Print and shaded views of the part. All mm, measured from the part's lowest x, y and z. A direction names the side the tool comes from. Give positions to 0.01 mm unless a question says otherwise; leave off trailing zeros. Loops run counter-clockwise (first coordinate to the right, second up) from the corner with the lowest first, then second, coordinate; pieces in that order, holes last. Notation, with made-up numbers: (84, -40) - (134, -40) arc R9 ccw to (134, -33) - close; hole circle Ø5 at (47, 54). An arc over 180 degrees is marked (long way). Return JSON: item names as keys, results as strings.
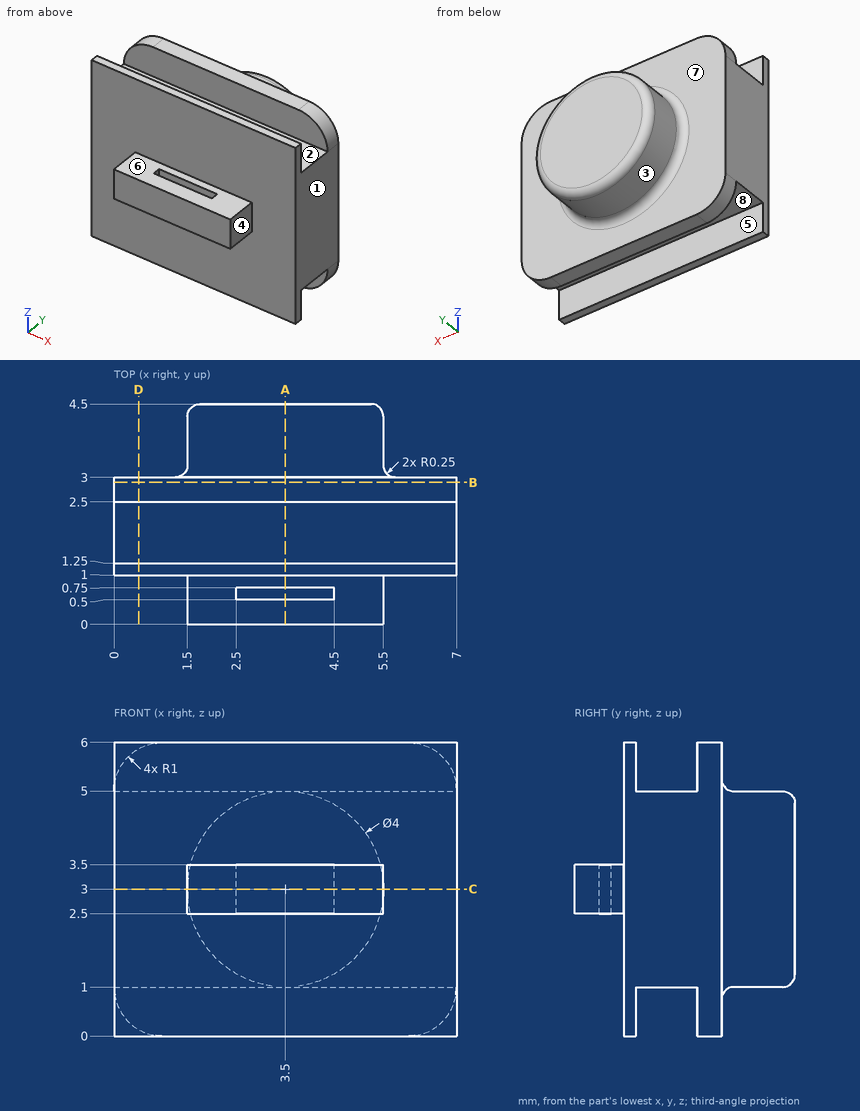
1. Drill centre lines: probe 1 along Y at (x, z) = (2.5, 5.45); probe 2 along Y at (x, z) = (4, 3); probe 3 along Y at (x, z) = (0.5, 1.8). Where is each one in solid material? Low to high.
Values follow:
{"probe 1": "y = 1 to 1.25, 2.5 to 3", "probe 2": "y = 0 to 0.5, 0.75 to 4.5", "probe 3": "y = 1 to 3"}
2. Drop flat-ended pins along their axis: P1, Ø0.8, axis at x = 2.5, y = 0.5, coming from the -Z side; P2, Ø0.8, axis at x = 3.5, y = 0.5, coming from the +Z side; P3, Ø0.5, axis at y = 0.5, z = 3, coming from the +X side. Give the stop position or say it passes through.
Values follow:
{"P1": "stops at z = 2.5", "P2": "stops at z = 3.5", "P3": "stops at x = 5.5"}
3. Which spindle directions (+Z, -Z, +X, -X, +Y, -Y) get a long thin tool onto all of the face, cutting with end or side? Do the marked faces 1, 2, 3, 4 and 5. Say none if no direction does.
Values follow:
{"face 1": "+Z, -Z, +X, +Y, -Y", "face 2": "+Z, +X, -X", "face 3": "+Y", "face 4": "+Z, -Z, +X, -Y", "face 5": "-Z, +X, -X"}
4. Cut at B-B, the plane y = 2.9. Write the cut outline in (x, z).
Values follow:
{"outline": "(0, 1) arc R1 ccw to (1, 0) - (6, 0) arc R1 ccw to (7, 1) - (7, 5) arc R1 ccw to (6, 6) - (1, 6) arc R1 ccw to (0, 5) - close"}
5. Cut at A-A, the plane x = 3.5. Write the cut outline in (y, z).
Values follow:
{"outline": "(0, 2.5) - (0.5, 2.5) - (0.5, 3.5) - (0, 3.5) - close; (0.75, 2.5) - (1, 2.5) - (1, 0) - (1.25, 0) - (1.25, 1) - (2.5, 1) - (2.5, 0) - (3, 0) - (3, 0.75) arc R0.25 cw to (3.25, 1) - (4.25, 1) arc R0.25 ccw to (4.5, 1.25) - (4.5, 4.75) arc R0.25 ccw to (4.25, 5) - (3.25, 5) arc R0.25 cw to (3, 5.25) - (3, 6) - (2.5, 6) - (2.5, 5) - (1.25, 5) - (1.25, 6) - (1, 6) - (1, 3.5) - (0.75, 3.5) - close"}
6. Cut at C-C, the plane z = 3. Write the cut outline in (x, y).
Values follow:
{"outline": "(0, 1) - (1.5, 1) - (1.5, 0) - (5.5, 0) - (5.5, 1) - (7, 1) - (7, 3) - (5.75, 3) arc R0.25 cw to (5.5, 3.25) - (5.5, 4.25) arc R0.25 ccw to (5.25, 4.5) - (1.75, 4.5) arc R0.25 ccw to (1.5, 4.25) - (1.5, 3.25) arc R0.25 cw to (1.25, 3) - (0, 3) - close; hole (2.5, 0.5) - (4.5, 0.5) - (4.5, 0.75) - (2.5, 0.75) - close"}
7. Pull direction Y, two halves, no side cores. Call the marked faces 6, 7 and 8: +Y half, -Y half, draft (parallel to the pull), parting line (faces both ways), or undercut.
Values follow:
{"face 6": "draft", "face 7": "+Y half", "face 8": "undercut"}
8. Cut at D-D, the plane x = 0.5. Write the cut outline in (y, z).
Values follow:
{"outline": "(1, 0) - (1.25, 0) - (1.25, 1) - (2.5, 1) - (2.5, 0.13) - (3, 0.13) - (3, 5.87) - (2.5, 5.87) - (2.5, 5) - (1.25, 5) - (1.25, 6) - (1, 6) - close"}
